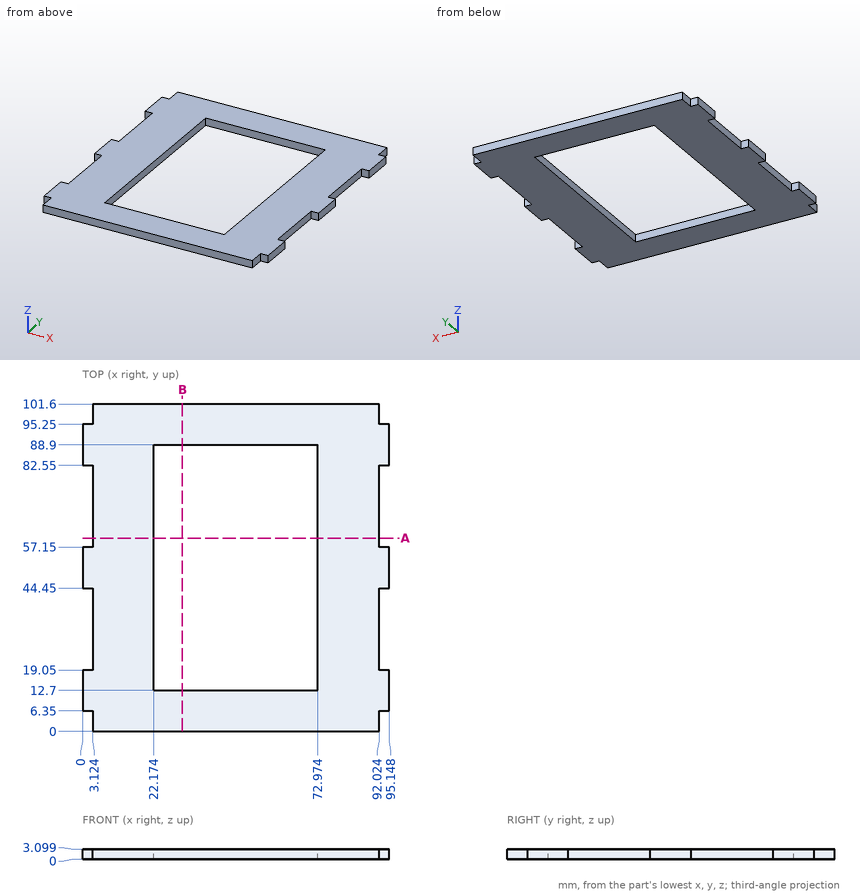
Can you work these out from the drawing? Everything is in mm from the part's minimum corner. Round coordinates to 2 decimals unless told otherwise and drop trailing zeros. Loops run counter-clockwise (first coordinate to the right, second up) from the corner with the lowest first, then second, coordinate; pieces in that order, holes last.
1. For P1, Ø1.5, axis at y = 30.5, z = 2, coming from the +X side; P2, Ø1.5, axis at x = 1.5, z = 1, coming from the +Y side; P3, Ø1.5, axis at y = 76, z = 2, coming from the -X side, each with a flat end and sliding along its axis, tell me the tip position at first contact or that it passes through.
Answer list:
P1: stops at x = 92.02
P2: stops at y = 95.25
P3: stops at x = 3.12
2. If we section it at B-B on x = 31: Write out the boundary of the cut face in (y, z).
Answer list:
outline: (0, 0) - (12.7, 0) - (12.7, 3.1) - (0, 3.1) - close; (88.9, 0) - (101.6, 0) - (101.6, 3.1) - (88.9, 3.1) - close
3. If I drill on line 1 along X through (y, z) = (72, 2.25) (1 decimal); line 2 along Y through (x, z) = (40.5, 1.5); line 3 along X through (y, z) = (17, 0.5) (1 decimal), over which ranges is the centre line in solid material (lowest first)?
Answer list:
line 1: x = 3.1 to 22.2, 73 to 92
line 2: y = 0 to 12.7, 88.9 to 101.6
line 3: x = 0 to 22.2, 73 to 95.1
4. If we section it at A-A on y = 60: Write out the boundary of the cut face in (x, z) (1 decimal).
Answer list:
outline: (3.1, 0) - (22.2, 0) - (22.2, 3.1) - (3.1, 3.1) - close; (73, 0) - (92, 0) - (92, 3.1) - (73, 3.1) - close
